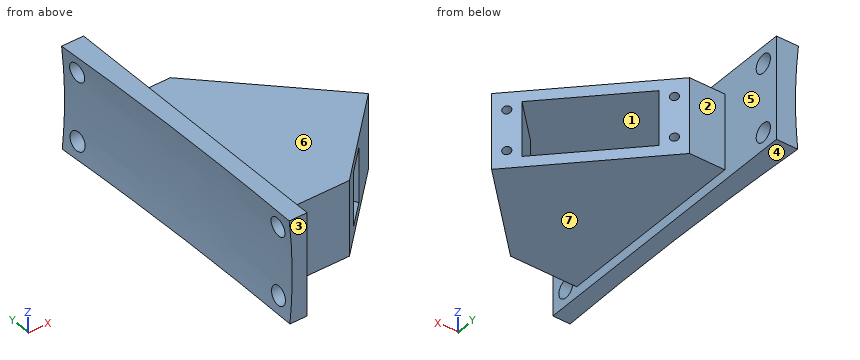
```python
from build123d import *

# Parameters (mm, degrees)
SKETCH1_W               = 15.24
SKETCH1_H               = 47.25
BOSS_EXTRUDE1_DEPTH     = 29
BOSS_EXTRUDE2_DEPTH     = 15.24
BOSS_EXTRUDE3_START     = 6.35
BOSS_EXTRUDE3_DEPTH     = 27.94
CUT_EXTRUDE4_DEPTH      = 90.856122335
CUT_EXTRUDE4_DEPTH_BACK = 90.856122335
BOSS_EXTRUDE4_START     = 12.7
SKETCH15_W              = 12.73404056
SKETCH15_H              = 107.95
BOSS_EXTRUDE4_DEPTH     = 38.1
SKETCH17_R              = 3.429
CUT_EXTRUDE6_DEPTH      = 95.762638832
BOSS_EXTRUDE9_DEPTH     = 6.35
BOSS_EXTRUDE10_DEPTH    = 6.35
SKETCH12_W              = 20.20062
SKETCH12_H              = 40.64
CUT_EXTRUDE8_DEPTH      = 38.1
SKETCH21_W              = 27.94
SKETCH21_H              = 50.342193805
CUT_EXTRUDE9_DEPTH      = 8
SKETCH22_W              = 27.94
SKETCH22_H              = 8
CUT_EXTRUDE10_DEPTH     = 2.54
BOSS_EXTRUDE11_DEPTH    = 13.97
SKETCH24_W              = 11.491520074
SKETCH24_H              = 20.20062
CUT_EXTRUDE11_DEPTH     = 112.502999945
SKETCH25_R              = 1.5
CUT_EXTRUDE12_DEPTH     = 18


with BuildPart() as part:
    # Sketch1 → Boss-Extrude1 (new body)
    with BuildSketch(Plane(origin=(0, 0, 0), x_dir=(0, 0, -1), z_dir=(1, 0, 0))):
        Rectangle(SKETCH1_W, SKETCH1_H)
    extrude(amount=BOSS_EXTRUDE1_DEPTH)

    # Sketch8 → Cut-Revolve1 (revolve, cut)
    with BuildSketch(Plane(origin=(0, 0, 0), x_dir=(1, 0, 0), z_dir=(0, 1, 0))):
        with BuildLine():
            Line((-1363.98, 509.27), (-1363.98, -509.27))
            add(Edge.make_bspline(
                [(-1363.98, -509.27), (8.89, -509.27), (8.89, 0), (8.89, 509.27), (-1363.98, 509.27)],
                knots=[4.71238898, 4.71238898, 4.71238898, 6.283185307, 6.283185307, 7.853981634, 7.853981634, 7.853981634], degree=2, weights=[1, 0.707106781, 1, 0.707106781, 1]))
        make_face()
    revolve(axis=Axis((-1363.98, 0, -509.27), (0, 0, 1)), mode=Mode.SUBTRACT)

    # Sketch9 → Boss-Extrude2 (add)
    with BuildSketch(Plane.XY.offset(7.62)):
        Polygon((29, -23.625), (57.293684645, -23.625), (29, 23.625), align=None)
    extrude(amount=-BOSS_EXTRUDE2_DEPTH)

    # Sketch11 → Boss-Extrude3 (add)
    with BuildSketch(Plane(origin=(0, 0, -7.62), x_dir=(-1, 0, 0), z_dir=(0, 0, -1)).offset(BOSS_EXTRUDE3_START)):
        Polygon((-8.532999942, 23.625), (-35.473768305, 50.565768363), (-71.071074924, 14.968461744), (-48.544371121, -9.013786608), (-28.889356272, 23.625), align=None)
    extrude(amount=-BOSS_EXTRUDE3_DEPTH)

    # Sketch13 → Cut-Extrude4 (cut, two sides: drawn at the far end of the back side and taken through both)
    with BuildSketch(Plane(origin=(0, 0, -7.62), x_dir=(-1, 0, 0), z_dir=(0, 0, -1)).offset(-CUT_EXTRUDE4_DEPTH_BACK)):
        Polygon((-61.672265147, 5.569651967), (-8.532999942, -23.625), (-25.02523354, -53.6436889), (-79.417056311, -23.760883228), align=None)
    extrude(amount=CUT_EXTRUDE4_DEPTH + CUT_EXTRUDE4_DEPTH_BACK, mode=Mode.SUBTRACT)

    # Sketch15 → Boss-Extrude4 (add)
    with BuildSketch(Plane.XY.offset(7.62).offset(BOSS_EXTRUDE4_START)):
        with Locations((7.499979662, 18.790026662)):
            Rectangle(SKETCH15_W, SKETCH15_H)
    extrude(amount=-BOSS_EXTRUDE4_DEPTH)

    # Sketch16 → Cut-Revolve2 (revolve, cut)
    with BuildSketch(Plane(origin=(0, 0, 0), x_dir=(1, 0, 0), z_dir=(0, 1, 0))):
        with BuildLine():
            Line((-1364.099005706, 509.27), (-1364.099005706, -509.27))
            add(Edge.make_bspline(
                [(-1364.099005706, -509.27), (8.770994294, -509.27), (8.770994294, 0), (8.770994294, 509.27), (-1364.099005706, 509.27)],
                knots=[4.71238898, 4.71238898, 4.71238898, 6.283185307, 6.283185307, 7.853981634, 7.853981634, 7.853981634], degree=2, weights=[1, 0.707106781, 1, 0.707106781, 1]))
        make_face()
    revolve(axis=Axis((-1364.099005706, 0, -509.27), (0, 0, 1)), mode=Mode.SUBTRACT)

    # Sketch17 → Cut-Extrude6 (cut, through all)
    with BuildSketch(Plane(origin=(13.866999942, 0, 0), x_dir=(0, 0, -1), z_dir=(1, 0, 0))):
        with Locations(Location((-13.97, -28.834973338, 0), (0, 0, 90))):
            Circle(SKETCH17_R)
        with Locations(Location((-13.97, 66.415026662, 0), (0, 0, 90))):
            Circle(SKETCH17_R)
        with Locations(Location((11.43, 66.415026662, 0), (0, 0, 90))):
            Circle(SKETCH17_R)
        with Locations(Location((11.43, -28.834973338, 0), (0, 0, 90))):
            Circle(SKETCH17_R)
    extrude(amount=-CUT_EXTRUDE6_DEPTH, mode=Mode.SUBTRACT)

    # Sketch19 → Boss-Extrude9 (add)
    with BuildSketch(Plane.XY.offset(7.62)):
        Polygon((13.866999942, 23.625), (13.866999942, -20.694506456), (45.209055073, -3.475216955), (28.889356272, 23.625), align=None)
    extrude(amount=BOSS_EXTRUDE9_DEPTH)

    # Sketch20 → Boss-Extrude10 (add)
    with BuildSketch(Plane(origin=(0, 0, -7.62), x_dir=(-1, 0, 0), z_dir=(0, 0, -1))):
        Polygon((-45.209055073, -3.475216955), (-13.866999942, -20.694506456), (-13.866999942, 23.625), (-28.889356272, 23.625), align=None)
    extrude(amount=BOSS_EXTRUDE10_DEPTH)

    # Sketch12 → Cut-Extrude8 (cut)
    with BuildSketch(Plane(origin=(43.019768334, 43.019768334, 0), x_dir=(0, 0, -1), z_dir=(0.7071067811865476, 0.7071067811865476, 0))):
        with Locations((0, -14.49944132)):
            Rectangle(SKETCH12_W, SKETCH12_H)
    extrude(amount=-CUT_EXTRUDE8_DEPTH, mode=Mode.SUBTRACT)

    # Sketch21 → Cut-Extrude9 (cut)
    with BuildSketch(Plane(origin=(43.019768334, 43.019768334, 0), x_dir=(0, 0, -1), z_dir=(0.7071067811865477, 0.7071067811865475, 0))):
        with Locations((0, -14.49944132)):
            Rectangle(SKETCH21_W, SKETCH21_H)
    extrude(amount=-CUT_EXTRUDE9_DEPTH, mode=Mode.SUBTRACT)

    # Sketch22 → Cut-Extrude10 (cut)
    with BuildSketch(Plane(origin=(28.05130659, -28.05130659, 0), x_dir=(0, 0, 1), z_dir=(-0.7071067811865476, 0.7071067811865476, 0))):
        with Locations((0, 56.839139829)):
            Rectangle(SKETCH22_W, SKETCH22_H)
    extrude(amount=-CUT_EXTRUDE10_DEPTH, mode=Mode.SUBTRACT)

    # Sketch23 → Boss-Extrude11 (add, symmetric)
    with BuildSketch(Plane.XY):
        Polygon((29.816914056, 44.908914114), (26.883196541, 47.842631629), (13.866999942, 47.842631629), (13.866999942, 28.959), align=None)
        Polygon((65.591257632, 9.134570538), (13.866999942, -20.694506456), (13.866999942, -23.674292513), (38.295755697, -23.674292513), (68.34793819, 6.37788998), align=None)
    extrude(amount=BOSS_EXTRUDE11_DEPTH, both=True)

    # Sketch24 → Cut-Extrude11 (cut, through all)
    with BuildSketch(Plane(origin=(12.416727049, -21.530870355, 0), x_dir=(0.8662714122168664, 0.49957365860881403, 0), z_dir=(-0.49957365860881403, 0.8662714122168664, 0))):
        with Locations((35.963054904, 0)):
            Rectangle(SKETCH24_W, SKETCH24_H)
    extrude(amount=-CUT_EXTRUDE11_DEPTH, mode=Mode.SUBTRACT)

    # Sketch25 → Cut-Extrude12 (cut)
    with BuildSketch(Plane(origin=(37.362914085, 37.362914085, 0), x_dir=(0, 0, -1), z_dir=(0.7071067811865476, 0.7071067811865475, 0))):
        with Locations(Location((-7.5, 10.32055868, 0), (0, 0, 90))):
            Circle(SKETCH25_R)
        with Locations(Location((7.5, 10.32055868, 0), (0, 0, 90))):
            Circle(SKETCH25_R)
        with Locations(Location((-7.5, -39.31944132, 0), (0, 0, 90))):
            Circle(SKETCH25_R)
        with Locations(Location((7.5, -39.31944132, 0), (0, 0, 90))):
            Circle(SKETCH25_R)
    extrude(amount=-CUT_EXTRUDE12_DEPTH, mode=Mode.SUBTRACT)


solid = part.part
```
The model under review builds one solid part; all positions refer to its coordinate system, in mm. Face numbers are marked on the shaded views. A direction names the side the tool comes from. Round coordinates to 2 decimals unless told otherwise and drop trailing zeros.
(1) For P1, Ø11, axis at y = 66.42, z = -11.43, coming from the +X side; P2, Ø6, axis at x = 38, z = -6.5, coming from the +Y side; P3, Ø3, axis at x = 38.5, y = 24.5, coming from the -Z side, all flat-tipped, find the tip position at first contact; note any pin that passes through.
Working result:
P1: stops at x = 13.87
P2: stops at y = -2.84
P3: stops at z = -13.97
(2) Tool access review of the marked faces 5, 6 and 7: name each direction out of +Z, -Z, +X, -X, +Y, -Y from which nothing blocks a thin tool from reaching the whole face with its end or side.
Working result:
face 5: +X
face 6: +Z, +X, +Y, -Y
face 7: -Z, +X, +Y, -Y
(3) Take a section at A-A, the plane z = -11.43. Count the separate pieces of the cut face and the enclosed holes in it, plus the area to 3 significant figures.
Working result:
separate pieces: 3
enclosed holes: 0
area: 3,140 mm2
(4) Mouldability with a two-part tool opening along Y and no side actions: class the marked faces 1, 2, 3 and 4 as released by +Y, released by -Y, zero draft, split by the parting line, or undercut.
Working result:
face 1: undercut
face 2: released by +Y
face 3: released by -Y
face 4: zero draft
(5) Wall thickness on L1, parallel to Y at x = 9.95, z = -11.43; L2, parallel to Z at x = 44, y = 3.5; L3, parallel to Z at x = 25.5, y = -15: over which ranges is each line inside the solid? List them lowest first.
Working result:
L1: y = -35.18 to -32.26, -25.41 to 62.99, 69.84 to 72.77
L2: z = -13.97 to -10.1, 10.1 to 13.97
L3: z = -13.97 to 13.97
